Autodesk Inventor part; units mm, degrees
ref_plane "YZ Plane" through (0, 0, 0) normal (1, 0, 0) x (0, 1, 0)
ref_plane "XZ Plane" through (0, 0, 0) normal (0, 1, 0) x (-1, 0, 0)
ref_plane "XY Plane" through (0, 0, 0) normal (0, 0, 1) x (1, 0, 0)
sketch "Sketch1" plane through (0, 0, 0) normal (0, 1, 0) x (-1, 0, 0)
  circle A0 centre (0, 0) radius 6.5
  dimension "d0" = 13
extrude "Extrusion1" add sketch "Sketch1" along normal blind 59
sketch "Sketch2" plane through (0, 59, 0) normal (0, 1, 0) x (1, 0, 0)
  circle A0 centre (0, 0) radius 6.5
  circle A1 centre (0, 0) radius 12
  dimension "d3" = 24
extrude "Extrusion2" add sketch "Sketch2" along normal blind 2 contours A0 | A1
sketch "Sketch3" plane through (0, 0, 0) normal (0, -1, 0) x (1, 0, 0)
  circle A0 centre (0, 0) radius 6.5
  circle A1 centre (0, 0) radius 12
  dimension "d6" = 24
extrude "Extrusion3" add sketch "Sketch3" along normal blind 2 contours A0 | A1
properties part number "Middle Arm Linkage"
Source: CAD feature listing. Evaluate the final solid. Frame: model axes, mm. A direction names the side the tool comes from. Coordinates: 2 decimals unless noted, no trailing zeros. Write each loop counter-clockwise with the first axis right and the second up, starting at its lowest first coordinate (ties: lowest second). Pieces come first, ordered by that corner, then holes. Notation, with made-up numbers: (24, 3) - (63, 3) arc R26 cw to (63, 35) - close; hole circle Ø11 at (-12.75, 53). An arc over 180 degrees is marked (long way). Answer as a JSON object with one key per item and string values.
Q1. Section query B-B, the plane x = 0. Output: boundary loops of the cut face in (y, z).
Ans:
{"outline": "(-2, -12) - (0, -12) - (0, -6.5) - (59, -6.5) - (59, -12) - (61, -12) - (61, 12) - (59, 12) - (59, 6.5) - (0, 6.5) - (0, 12) - (-2, 12) - close"}
Q2. Set-up query: faces 1 (the flat face through (0, 61, 0)), 2 (the flat face through (5, 59, 5)). Return all of +Z, -Z, +X, -X, +Y, -Y with unobstructed straight access to the full face (end or side cutting, diameter ignored); none if empty.
Ans:
{"face 1": "+Z, -Z, +X, -X, +Y", "face 2": "none"}
Q3. Section query C-C, the plane z = 0. Output: boundary loops of the cut face in (x, y), plus the area to 3 significant figures.
Ans:
{"outline": "(-12, -2) - (12, -2) - (12, 0) - (6.5, 0) - (6.5, 59) - (12, 59) - (12, 61) - (-12, 61) - (-12, 59) - (-6.5, 59) - (-6.5, 0) - (-12, 0) - close", "area": "863 mm2"}
Q4. Material intervals for line 1 (Y direction, x = -4.5, z = -9); line 2 (X direction, y = 45, z = -0.25); line 3 (Z direction, x = 4.75, y = 9), sorted ascending. Write a range as [from, to].
Ans:
{"line 1": "y = [-2, 0], [59, 61]", "line 2": "x = [-6.5, 6.5]", "line 3": "z = [-4.44, 4.44]"}
Q5. First-contact query: pin 1 Ø12 at (x, y) = (6, 50.5) entering from +Z; pin 2 Ø4 at (y, z) = (5, 1.5) entering from +X; pin 3 Ø1.5 at (x, y) = (3, 14.5) entering from +Z. Flat tips, straight axial feed; report the tip coordinate or a pass-through.
Ans:
{"pin 1": "stops at z = 6.5", "pin 2": "stops at x = 6.5", "pin 3": "stops at z = 6.1"}
Q6. Draft query along Y for faces 3 (the flat face through (0, -2, 0)), 4 (the cylindrical face through (-11.99, 59.99, 0.53)), 5 (the cylindrical face through (5.158, 29.087, 3.955)). Return one class per face: released by +Y, released by -Y, zero draft, split by the parting line, or undercut.
Ans:
{"face 3": "released by -Y", "face 4": "zero draft", "face 5": "undercut"}
Q7. Section query A-A, the plane z = 10.25. Output: boundary loops of the cut face in (x, y), plus the area to 3 significant figures.
Ans:
{"outline": "(-6.24, -2) - (6.24, -2) - (6.24, 0) - (-6.24, 0) - close; (-6.24, 59) - (6.24, 59) - (6.24, 61) - (-6.24, 61) - close", "area": "49.9 mm2"}
Q8. Section query D-D, the plane y = 26. Output: boundary loops of the cut face in (x, z), plus the area to 3 significant figures.
Ans:
{"outline": "circle Ø13 at (0, 0)", "area": "133 mm2"}
